from build123d import *

# Parameters (mm, degrees)
SKETCH_1_R               = 44.95
SKETCH_1_R_2             = 2.5
SKETCH_1_R_3             = 18.4
EXTRUDE_1_DEPTH          = 16
SKETCH_2_R               = 4
CUT_EXTRUDE_1_DEPTH      = 3
SKETCH_4_R               = 4.5
CUT_EXTRUDE_2_DEPTH      = 5.1
SKETCH_5_R               = 1.5
CUT_EXTRUDE_3_DEPTH      = 10
PATTERN_CIRCULAR_1_COUNT = 12
FILLET_1_R               = 0.5


with BuildPart() as part:
    # 草图1 → 凸台-拉伸1 (new body)
    with BuildSketch(Plane(origin=(0, 0, 0), x_dir=(1, 0, 0), z_dir=(0, 1, 0))):
        Circle(SKETCH_1_R)
        with Locations((-24.6, 0)):
            Circle(SKETCH_1_R_2, mode=Mode.SUBTRACT)
        with Locations((-12.3, 21.304224933)):
            Circle(SKETCH_1_R_2, mode=Mode.SUBTRACT)
        with Locations((12.3, 21.304224933)):
            Circle(SKETCH_1_R_2, mode=Mode.SUBTRACT)
        with Locations((24.6, 0)):
            Circle(SKETCH_1_R_2, mode=Mode.SUBTRACT)
        with Locations((12.3, -21.304224933)):
            Circle(SKETCH_1_R_2, mode=Mode.SUBTRACT)
        with Locations((-12.3, -21.304224933)):
            Circle(SKETCH_1_R_2, mode=Mode.SUBTRACT)
        Circle(SKETCH_1_R_3, mode=Mode.SUBTRACT)
    extrude(amount=EXTRUDE_1_DEPTH)

    # 草图2 → 切除-拉伸1 (cut)
    with BuildSketch(Plane.XZ):
        with Locations((-21.304224933, -12.3)):
            Circle(SKETCH_2_R)
        with Locations((0, 24.6)):
            Circle(SKETCH_2_R)
        with Locations((21.304224933, -12.3)):
            Circle(SKETCH_2_R)
    extrude(amount=-CUT_EXTRUDE_1_DEPTH, mode=Mode.SUBTRACT)

    # 草图4 → 切除-拉伸2 (cut)
    with BuildSketch(Plane(origin=(0, 16, 0), x_dir=(1, 0, 0), z_dir=(0, 1, 0))):
        with Locations((-24.6, 0)):
            Circle(SKETCH_4_R)
        with Locations((-12.3, 21.304224933)):
            Circle(SKETCH_4_R)
        with Locations((12.3, 21.304224933)):
            Circle(SKETCH_4_R)
        with Locations((24.6, 0)):
            Circle(SKETCH_4_R)
        with Locations((12.3, -21.304224933)):
            Circle(SKETCH_4_R)
        with Locations((-12.3, -21.304224933)):
            Circle(SKETCH_4_R)
    extrude(amount=-CUT_EXTRUDE_2_DEPTH, mode=Mode.SUBTRACT)

    # 草图5 → 切除-拉伸3 (cut)
    with BuildSketch(Plane(origin=(43, 0, 0), x_dir=(0, 0, -1), z_dir=(1, 0, 0))):
        with Locations((0, 12)):
            Circle(SKETCH_5_R)
    cut_extrude_3 = extrude(amount=-CUT_EXTRUDE_3_DEPTH, mode=Mode.SUBTRACT)

    # 阵列(圆周)1: 切除-拉伸3 ×12 about axis
    pattern_circular_1_axis = Axis((0, 0, 0), (0, 1, 0))
    for i in range(1, PATTERN_CIRCULAR_1_COUNT):
        add(cut_extrude_3.rotate(pattern_circular_1_axis, i * 360 / PATTERN_CIRCULAR_1_COUNT), mode=Mode.SUBTRACT)

    # 圆角1
    fillet_1_edges = [part.edges().sort_by_distance(p)[0] for p in [
        (-18.4, 16, 0),
    ]]
    fillet(fillet_1_edges, radius=FILLET_1_R)


solid = part.part
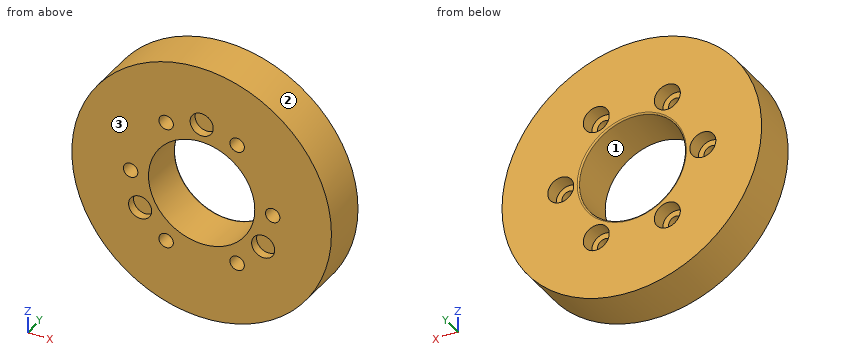
For this review, take the finished solid that the model builds, in its own axes (mm). Face numbers are marked on the shaded views. Round coordinates to 2 decimals unless told otherwise and drop trailing zeros. Loops run counter-clockwise (first coordinate to the right, second up) from the corner with the lowest first, then second, coordinate; pieces in that order, holes last. Notation, with made-up numbers: (50, 60) - (100, 60) arc R23 cw to (100, 88) - close; hole circle Ø1 at (81.5, -31). An arc over 180 degrees is marked (long way). Use one line per item in the form item = value.
1) Mouldability with a two-part tool opening along Z and no side actions: class the marked faces 1, 2 and 3 as pulls with the +Z half, pulls with the -Z half, needs draft (parallel to the pull), parting line crosses it, or undercut.
Solutions:
face_1 = undercut
face_2 = parting line crosses it
face_3 = needs draft
2) We need section B-B on x = 0. Write out the cut boundary in (y, z).
Solutions:
outline = (0, -44.95) - (16, -44.95) - (16, -18.9) arc R0.5 ccw to (15.5, -18.4) - (0, -18.4) - close; (0, 18.4) - (15.5, 18.4) arc R0.5 ccw to (16, 18.9) - (16, 44.95) - (0, 44.95) - (0, 28.6) - (3, 28.6) - (3, 20.6) - (0, 20.6) - close; hole (10.5, -43) - (13.5, -43) - (13.5, -33) - (10.5, -33) - close; hole (10.5, 33) - (13.5, 33) - (13.5, 43) - (10.5, 43) - close
3) We need section C-C on y = 5.5. Write out the cut boundary in (x, z).
Solutions:
outline = circle Ø89.9 at (0, 0); hole circle Ø5 at (-24.6, 0); hole circle Ø36.8 at (0, 0); hole circle Ø5 at (-12.3, -21.3); hole circle Ø5 at (-12.3, 21.3); hole circle Ø5 at (12.3, -21.3); hole circle Ø5 at (12.3, 21.3); hole circle Ø5 at (24.6, 0)
4) Clearance check with flat-ended pins moving along their axes: P1, Ø5, axis at x = 0, z = 24.6, coming from the -Y side; P2, Ø6, axis at y = 13.5, z = -16.5, coming from the -X side; P3, Ø7, axis at x = -24.6, z = 0, coming from the +Y side. State where each tip first meets the part, or that it passes through.
Solutions:
P1 = 3
P2 = -42.87
P3 = 10.9
5) We need section A-A on z = 0. State how many separate pieces and enclosed holes the cut face has, then the cut area to 3 significant figures.
Solutions:
separate_pieces = 4
enclosed_holes = 2
area = 589 mm2
6) Wall thickness on probe 1 along X at (y, z) = (5, 0); probe 2 along Z at (x, y) = (-11.5, 3); probe 3 along X at (y, z) = (14, 0): over which ranges is each line inside the solid? List them lowest first.
Solutions:
probe_1 = -44.95 to -27.1, -22.1 to -18.4, 18.4 to 22.1, 27.1 to 44.95
probe_2 = -43.45 to -23.67, -18.94 to -14.36, 14.36 to 18.94, 23.67 to 43.45
probe_3 = -44.95 to -29.1, -20.1 to -18.4, 18.4 to 20.1, 29.1 to 44.95
